```python
from build123d import *

# Parameters (mm, degrees)
F0_W     = 76.2
F0_H     = 19.05
F1_DEPTH = 19.05
F3_D     = 12.7
F4_R     = 6.35
F5_DEPTH = 51.054


with BuildPart() as f1:
    # F0 (on Top) → F1 (new body)
    with BuildSketch(Plane.XY):
        with Locations((9.621889, -4.491718)):
            Rectangle(F0_W, F0_H)
    extrude(amount=F1_DEPTH)

    # F3 (through all)
    with Locations(Plane(origin=(0, 5.033282, 0), x_dir=(-1, 0, 0), z_dir=(0, 1, 0))):
        with Locations((18.953111, 9.525)):
            Hole(F3_D / 2)

    # F4 (on face) → F5 (cut)
    with BuildSketch(Plane.XZ.offset(14.016718)):
        with Locations((38.593322, 9.200889)):
            Circle(F4_R)
    extrude(amount=-F5_DEPTH, mode=Mode.SUBTRACT)


solid = f1.part
```
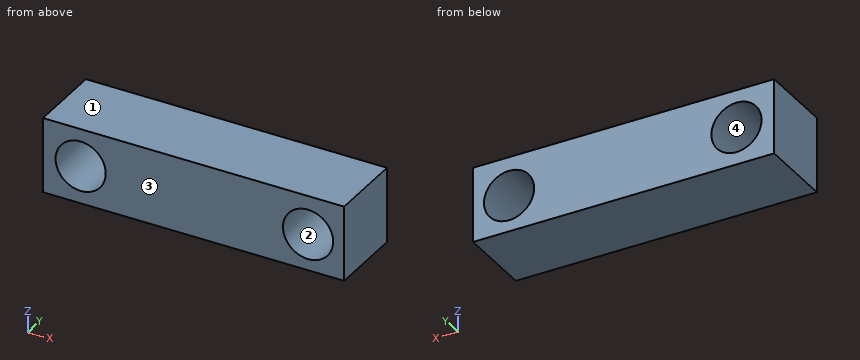
Here's how the part is built. I have some questions about the finished solid (model axes, mm). Face numbers are marked on the shaded views. Coordinates: 2 decimals unless noted, no trailing zeros. Write each loop counter-clockwise with the first axis right and the second up, starting at its lowest first coordinate (ties: lowest second). Pieces come first, ordered by that corner, then holes. Notation, with made-up numbers: (50, 11.5) -> (98, 11.5) arc R28 cw to (98, 43.5) -> close; hole circle Ø6 at (79, 13). An arc over 180 degrees is marked (long way). Use a Markdown table: item, result. Add a question column.
(1) If we section it at D-D, the plane x = 42: Write out the boundary of the cut face in (y, z).
(2) If we section it at C-C, the plane y = -3.5: Write out the boundary of the cut face in (x, z) (3 decimals), and give its area (3 significant figures).
(3) Please list where these lines run through material, in increasing order: line 1 (X direction, y = 0.5, z = 9.5); line 2 (X direction, y = -12.5, z = 12.75); line 3 (Z direction, x = -18.5, y = -1.75).
(4) If we section it at B-B, the plane x = -19: Write out the boundary of the cut face in (y, z), and give its area (3 significant figures).
(5) If we section it at A-A, the plane z = 11.75: Write out the boundary of the cut face in (x, y), and give its area (3 significant figures).
(6) We'd pull the mould along Z, two halves only. Please class the marked faces 1, 2, 3 and 4: +Z half, -Z half, draft (parallel to the pull), parting line (faces both ways), or undercut.
Outcome:
| question | item | result |
|---|---|---|
| 1 | outline | (-14.02, 0) -> (5.03, 0) -> (5.03, 3.84) -> (-14.02, 3.84) -> close; (-14.02, 14.56) -> (5.03, 14.56) -> (5.03, 19.05) -> (-14.02, 19.05) -> close |
| 2 | outline | (-28.478, 0) -> (47.722, 0) -> (47.722, 19.05) -> (-28.478, 19.05) -> close; hole circle Ø12.7 at (-18.953, 9.525); hole circle Ø12.7 at (38.593, 9.201) |
| 2 | area | 1,200 mm^2 |
| 3 | line 1 | x = -28.48 to -25.3, -12.6 to 32.25, 44.94 to 47.72 |
| 3 | line 2 | x = -28.48 to -24.42, -13.48 to 33.33, 43.86 to 47.72 |
| 3 | line 3 | z = 0 to 3.19, 15.86 to 19.05 |
| 4 | outline | (-14.02, 0) -> (5.03, 0) -> (5.03, 3.18) -> (-14.02, 3.18) -> close; (-14.02, 15.87) -> (5.03, 15.87) -> (5.03, 19.05) -> (-14.02, 19.05) -> close |
| 4 | area | 121 mm^2 |
| 5 | outline | (-28.48, -14.02) -> (-24.9, -14.02) -> (-24.9, 5.03) -> (-28.48, 5.03) -> close; (-13.01, -14.02) -> (32.78, -14.02) -> (32.78, 5.03) -> (-13.01, 5.03) -> close; (44.41, -14.02) -> (47.72, -14.02) -> (47.72, 5.03) -> (44.41, 5.03) -> close |
| 5 | area | 1,000 mm^2 |
| 6 | face 1 | +Z half |
| 6 | face 2 | undercut |
| 6 | face 3 | draft |
| 6 | face 4 | undercut |
